from build123d import *

# Parameters (mm, degrees)
SKETCH1_W                 = 17.78
SKETCH1_H                 = 74.93
BOSS_EXTRUDE1_DEPTH       = 12.7
CUT_EXTRUDE1_DEPTH        = 10.16
TAP_DRILL_FOR_6_32_TAP1_D = 2.7051
SKETCH5_R                 = 2.36855
CUT_EXTRUDE2_DEPTH        = 11.1125


with BuildPart() as part:
    # Sketch1 → Boss-Extrude1 (new body)
    with BuildSketch(Plane(origin=(0, 0, 0), x_dir=(0, 0, -1), z_dir=(1, 0, 0))):
        with Locations((8.89, 37.465)):
            Rectangle(SKETCH1_W, SKETCH1_H)
    extrude(amount=BOSS_EXTRUDE1_DEPTH)

    # Sketch2 → Cut-Extrude1 (cut)
    with BuildSketch(Plane(origin=(12.7, 0, 0), x_dir=(0, 0, -1), z_dir=(1, 0, 0))):
        Polygon((0, 64.77), (10.16, 64.77), (13.97, 64.77), (24.13, 64.77), (24.13, 10.16), (13.97, 10.16), (10.16, 10.16), (0, 10.16), align=None)
    extrude(amount=-CUT_EXTRUDE1_DEPTH, mode=Mode.SUBTRACT)

    # Tap Drill for #6-32 Tap1 (through all)
    with Locations(Plane(origin=(12.7, 0, 0), x_dir=(0, 0, -1), z_dir=(1, 0, 0))):
        with Locations((5.08, 69.85), (5.08, 5.08)):
            Hole(TAP_DRILL_FOR_6_32_TAP1_D / 2)

    # Sketch5 → Cut-Extrude2 (cut)
    with BuildSketch(Plane(origin=(0, 0, -17.78), x_dir=(-1, 0, 0), z_dir=(0, 0, -1))):
        with Locations((-6.35, 69.85)):
            Circle(SKETCH5_R)
        with Locations((-6.35, 5.08)):
            Circle(SKETCH5_R)
    extrude(amount=-CUT_EXTRUDE2_DEPTH, mode=Mode.SUBTRACT)


solid = part.part
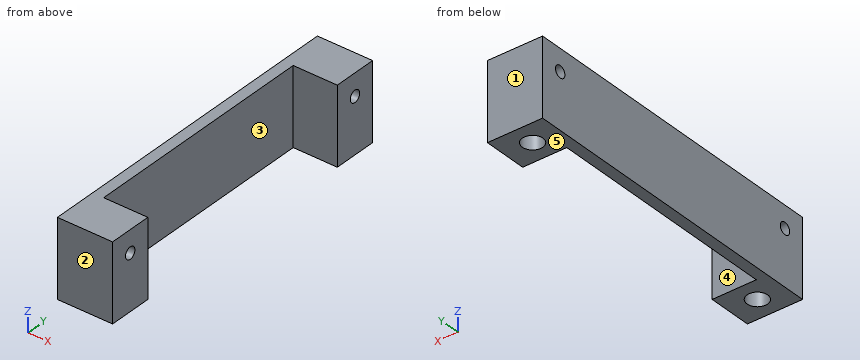
Verification items for the finished model (mm, model axes). Face numbers are marked on the shaded views. A direction names the side the tool comes from. Give positions to 0.01 mm unless a question says otherwise; leave off trailing zeros. Loops run counter-clockwise (first coordinate to the right, second up) from the corner with the lowest first, then second, coordinate; pieces in that order, holes last.
1) Depth check by flat-ended pin: pin 1 Ø9 at (y, z) = (40, -11) entering from +X; pin 2 Ø2.5 at (x, y) = (6, 5) entering from -Z. Enter the tip coordinate at first touch or a pass-through.
2) Set-up check for the marked faces 4 and 5: record each of +Z, -Z, +X, -X, +Y, -Y from which the full face is reachable in a straight line by a thin tool's end or side.
3) Sectioned sample at A-A, the plane x = 6.35. Enter the section's corners in (y, z), then the cut area to 3 significant figures.
4) Thickness scan on line 1 along Y through (x, z) = (4.25, -5.08); line 2 along Y through (x, z) = (6.35, -13.5); line 3 along Y through (x, z) = (1, -4.75). Record the ranges inside material, lowest first.
5) Sectioned sample at D-D, the plane z = -10.25. Enter the section's corners in (x, y).
6) Sectioned sample at B-B, the plane z = -5.08. Enter the section's corners in (x, y), then the cut area to 3 significant figures.
7) Sectioned sample at C-C, the plane y = 5.08. Enter the section's corners in (x, z).
8) Draft check along Y on the marked faces 1, 2 and 3. Enter one of: pulls with the +Y half, pulls with the -Y half, needs draft (parallel to the pull), parting line crosses it, or undercut.
Answers:
1. pin 1: stops at x = 2.54
1. pin 2: stops at z = -6.67
2. face 4: +Z, -Z, +X
2. face 5: -Z, +X, -X, +Y, -Y
3. outline: (0, -17.78) - (2.71, -17.78) - (2.71, -6.67) - (7.45, -6.67) - (7.45, -17.78) - (10.16, -17.78) - (10.16, 0) - (0, 0) - close; (64.77, -17.78) - (67.48, -17.78) - (67.48, -6.67) - (72.22, -6.67) - (72.22, -17.78) - (74.93, -17.78) - (74.93, 0) - (64.77, 0) - close; hole circle Ø2.71 at (5.08, -5.08); hole circle Ø2.71 at (69.85, -5.08)
3. area: 245 mm2
4. line 1: y = 0 to 3.73, 6.43 to 10.16, 64.77 to 68.5, 71.2 to 74.93
4. line 2: y = 0 to 2.71, 7.45 to 10.16, 64.77 to 67.48, 72.22 to 74.93
4. line 3: y = 0 to 3.77, 6.39 to 68.54, 71.16 to 74.93
5. outline: (0, 0) - (12.7, 0) - (12.7, 10.16) - (2.54, 10.16) - (2.54, 64.77) - (12.7, 64.77) - (12.7, 74.93) - (0, 74.93) - close; hole circle Ø4.74 at (6.35, 5.08); hole circle Ø4.74 at (6.35, 69.85)
6. outline: (0, 0) - (12.7, 0) - (12.7, 3.73) - (0, 3.73) - close; (0, 6.43) - (12.7, 6.43) - (12.7, 10.16) - (2.54, 10.16) - (2.54, 64.77) - (12.7, 64.77) - (12.7, 68.5) - (0, 68.5) - close; (0, 71.2) - (12.7, 71.2) - (12.7, 74.93) - (0, 74.93) - close
6. area: 328 mm2
7. outline: (0, -17.78) - (3.98, -17.78) - (3.98, -6.67) - (8.72, -6.67) - (8.72, -17.78) - (12.7, -17.78) - (12.7, -6.43) - (0, -6.43) - close; (0, -3.73) - (12.7, -3.73) - (12.7, 0) - (0, 0) - close
8. face 1: pulls with the +Y half
8. face 2: pulls with the -Y half
8. face 3: undercut
